Can you work these out from the model? Positions are in its coordinate system, mm. Give positions to 0.01 mm unless a question says otherwise; leave off trailing zeros. Order: outer loops, then holes, each group sorted by start corner. A loop starts at its lowest first (then second) coordinate and runs counter-clockwise, first axis right, second up. Notation, with made-up numbers: (41.25, -16.5) - (75.25, -16.5) arc R24 ccw to (75.25, -6.5) - close; hole circle Ø8 at (-37, -21). An arc over 180 degrees is marked (long way). One line per question, with ' | ' between items.
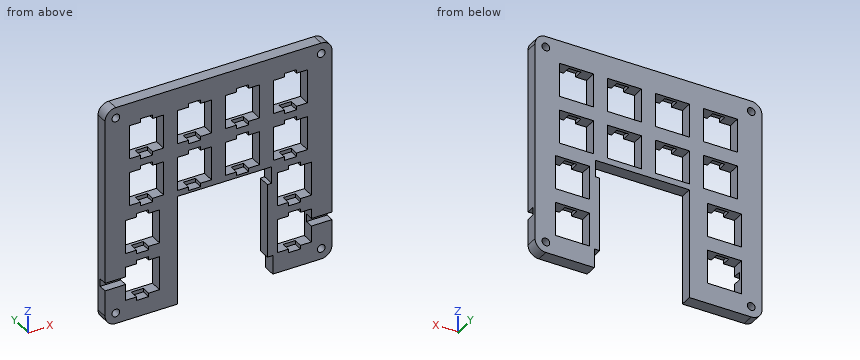
```python
from build123d import *

# Parameters (mm, degrees)
SKETCH2_R           = 1.6
BOSS_EXTRUDE1_DEPTH = 5
CUT_EXTRUDE1_DEPTH  = 3.5
SKETCH4_W           = 2.5
SKETCH4_H           = 1.5
CUT_EXTRUDE2_DEPTH  = 3.7


with BuildPart() as part:
    # Sketch2 → Boss-Extrude1 (new body)
    with BuildSketch(Plane(origin=(0, 0, 0), x_dir=(1, 0, 0), z_dir=(0, 1, 0))):
        with BuildLine():
            Line((-46.858540632, -41.275), (-46.858540632, 41.275))
            ThreePointArc((-46.858540632, 41.275), (-45.557936393, 44.414936393), (-42.418, 45.715540632))
            Line((-42.418, 45.715540632), (-16.875382857, 45.715540632))
            Line((-16.875382857, 45.715540632), (-16.875382857, 30.218907102))
            Line((-16.875382857, 30.218907102), (-16.875382857, 0.094907102))
            Line((-16.875382857, 0.094907102), (-9.912382857, 0.094907102))
            Line((-9.912382857, 0.094907102), (21.96872062, 0.094907102))
            Line((21.96872062, 0.094907102), (21.96872062, 7.075))
            Line((21.96872062, 7.075), (20.16872062, 7.075))
            Line((20.16872062, 7.075), (20.16872062, 9.575))
            Line((20.16872062, 9.575), (20.16872062, 37.797317828))
            Line((20.16872062, 37.797317828), (22.418, 37.797317828))
            Line((22.418, 37.797317828), (22.418, 39.575))
            Line((22.418, 39.575), (22.418, 41.275))
            Line((22.418, 41.275), (22.418, 45.715540632))
            Line((22.418, 45.715540632), (42.418, 45.715540632))
            ThreePointArc((42.418, 45.715540632), (45.557936393, 44.414936393), (46.858540632, 41.275))
            Line((46.858540632, 41.275), (46.858540632, -41.275))
            ThreePointArc((46.858540632, -41.275), (45.557936393, -44.414936393), (42.418, -45.715540632))
            Line((42.418, -45.715540632), (-42.418, -45.715540632))
            ThreePointArc((-42.418, -45.715540632), (-45.557936393, -44.414936393), (-46.858540632, -41.275))
        make_face()
        with Locations(Location((42.418, 41.275, 0), (0, 0, 270))):
            Circle(SKETCH2_R, mode=Mode.SUBTRACT)
        with Locations(Location((-42.418, 41.275, 0), (0, 0, 270))):
            Circle(SKETCH2_R, mode=Mode.SUBTRACT)
        with Locations(Location((-42.418, -41.275, 0), (0, 0, 270))):
            Circle(SKETCH2_R, mode=Mode.SUBTRACT)
        with Locations(Location((42.418, -41.275, 0), (0, 0, 270))):
            Circle(SKETCH2_R, mode=Mode.SUBTRACT)
        Polygon((-31.375382857, 37.218907102), (-38.375382857, 37.218907102), (-38.375382857, 23.218907102), (-24.375382857, 23.218907102), (-24.375382857, 37.218907102), align=None, mode=Mode.SUBTRACT)
        Polygon((-38.375382857, 10.406907102), (-38.375382857, 17.406907102), (-24.375382857, 17.406907102), (-24.375382857, 3.406907102), (-38.375382857, 3.406907102), align=None, mode=Mode.SUBTRACT)
        Polygon((-36.724382857, -9.405092898), (-36.724382857, -2.405092898), (-22.724382857, -2.405092898), (-22.724382857, -16.405092898), (-36.724382857, -16.405092898), align=None, mode=Mode.SUBTRACT)
        Polygon((-36.724382857, -29.217092898), (-36.724382857, -22.217092898), (-22.724382857, -22.217092898), (-22.724382857, -36.217092898), (-36.724382857, -36.217092898), align=None, mode=Mode.SUBTRACT)
        Polygon((-9.912382857, -22.217092898), (-2.912382857, -22.217092898), (-2.912382857, -36.217092898), (-16.912382857, -36.217092898), (-16.912382857, -22.217092898), align=None, mode=Mode.SUBTRACT)
        Polygon((-9.912382857, -16.405092898), (-2.912382857, -16.405092898), (-2.912382857, -2.405092898), (-16.912382857, -2.405092898), (-16.912382857, -16.405092898), align=None, mode=Mode.SUBTRACT)
        Polygon((9.899617143, -2.405092898), (2.899617143, -2.405092898), (2.899617143, -16.405092898), (16.899617143, -16.405092898), (16.899617143, -2.405092898), align=None, mode=Mode.SUBTRACT)
        Polygon((9.899617143, -22.217092898), (2.899617143, -22.217092898), (2.899617143, -36.217092898), (16.899617143, -36.217092898), (16.899617143, -22.217092898), align=None, mode=Mode.SUBTRACT)
        Polygon((36.711617143, -29.217092898), (36.711617143, -22.217092898), (22.711617143, -22.217092898), (22.711617143, -36.217092898), (36.711617143, -36.217092898), align=None, mode=Mode.SUBTRACT)
        Polygon((29.711617143, -2.405092898), (22.711617143, -2.405092898), (22.711617143, -16.405092898), (36.711617143, -16.405092898), (36.711617143, -2.405092898), align=None, mode=Mode.SUBTRACT)
        Polygon((38.362617143, 10.406907102), (38.362617143, 17.406907102), (24.362617143, 17.406907102), (24.362617143, 3.406907102), (38.362617143, 3.406907102), align=None, mode=Mode.SUBTRACT)
        Polygon((38.362617143, 30.218907102), (38.362617143, 23.218907102), (24.362617143, 23.218907102), (24.362617143, 37.218907102), (38.362617143, 37.218907102), align=None, mode=Mode.SUBTRACT)
    extrude(amount=BOSS_EXTRUDE1_DEPTH)

    # Sketch3 → Cut-Extrude1 (cut)
    with BuildSketch(Plane.XZ):
        Polygon((38.362617143, -30.492), (42.418, -30.492), (46.218, -30.492), (46.858540632, -30.492), (46.858540632, -27.292), (46.218, -27.292), (38.362617143, -27.292), align=None)
        Polygon((-46.218, -27.292), (-46.858540632, -27.292), (-46.858540632, -30.492), (-46.218, -30.492), (-42.418, -30.492), (-38.375382857, -30.492), (-38.375382857, -27.292), align=None)
    extrude(amount=-CUT_EXTRUDE1_DEPTH, mode=Mode.SUBTRACT)

    # Sketch4 → Cut-Extrude2 (cut)
    with BuildSketch(Plane.XZ):
        with Locations((32.612617143, -37.968907102)):
            Rectangle(SKETCH4_W, SKETCH4_H)
        with Locations((30.112617143, -37.968907102)):
            Rectangle(SKETCH4_W, SKETCH4_H)
        with Locations((32.612617143, -22.468907102)):
            Rectangle(SKETCH4_W, SKETCH4_H)
        with Locations((30.112617143, -22.468907102)):
            Rectangle(SKETCH4_W, SKETCH4_H)
        with Locations((32.612617143, -2.656907102)):
            Rectangle(SKETCH4_W, SKETCH4_H)
        with Locations((30.112617143, -18.156907102)):
            Rectangle(SKETCH4_W, SKETCH4_H)
        with Locations((32.612617143, -18.156907102)):
            Rectangle(SKETCH4_W, SKETCH4_H)
        with Locations((30.112617143, -2.656907102)):
            Rectangle(SKETCH4_W, SKETCH4_H)
        with Locations((30.961617143, 1.655092898)):
            Rectangle(SKETCH4_W, SKETCH4_H)
        with Locations((28.461617143, 1.655092898)):
            Rectangle(SKETCH4_W, SKETCH4_H)
        with Locations((30.961617143, 17.155092898)):
            Rectangle(SKETCH4_W, SKETCH4_H)
        with Locations((28.461617143, 17.155092898)):
            Rectangle(SKETCH4_W, SKETCH4_H)
        with Locations((30.961617143, 21.467092898)):
            Rectangle(SKETCH4_W, SKETCH4_H)
        with Locations((28.461617143, 21.467092898)):
            Rectangle(SKETCH4_W, SKETCH4_H)
        with Locations((30.961617143, 36.967092898)):
            Rectangle(SKETCH4_W, SKETCH4_H)
        with Locations((28.461617143, 36.967092898)):
            Rectangle(SKETCH4_W, SKETCH4_H)
        with Locations((11.149617143, 36.967092898)):
            Rectangle(SKETCH4_W, SKETCH4_H)
        with Locations((8.649617143, 36.967092898)):
            Rectangle(SKETCH4_W, SKETCH4_H)
        with Locations((8.649617143, 21.467092898)):
            Rectangle(SKETCH4_W, SKETCH4_H)
        with Locations((11.149617143, 21.467092898)):
            Rectangle(SKETCH4_W, SKETCH4_H)
        with Locations((11.149617143, 17.155092898)):
            Rectangle(SKETCH4_W, SKETCH4_H)
        with Locations((8.649617143, 17.155092898)):
            Rectangle(SKETCH4_W, SKETCH4_H)
        with Locations((11.149617143, 1.655092898)):
            Rectangle(SKETCH4_W, SKETCH4_H)
        with Locations((8.649617143, 1.655092898)):
            Rectangle(SKETCH4_W, SKETCH4_H)
        with Locations((-8.662382857, 1.655092898)):
            Rectangle(SKETCH4_W, SKETCH4_H)
        with Locations((-11.162382857, 1.655092898)):
            Rectangle(SKETCH4_W, SKETCH4_H)
        with Locations((-8.662382857, 17.155092898)):
            Rectangle(SKETCH4_W, SKETCH4_H)
        with Locations((-11.162382857, 17.155092898)):
            Rectangle(SKETCH4_W, SKETCH4_H)
        with Locations((-8.662382857, 21.467092898)):
            Rectangle(SKETCH4_W, SKETCH4_H)
        with Locations((-11.162382857, 21.467092898)):
            Rectangle(SKETCH4_W, SKETCH4_H)
        with Locations((-8.662382857, 36.967092898)):
            Rectangle(SKETCH4_W, SKETCH4_H)
        with Locations((-11.162382857, 36.967092898)):
            Rectangle(SKETCH4_W, SKETCH4_H)
        with Locations((-28.474382857, 17.155092898)):
            Rectangle(SKETCH4_W, SKETCH4_H)
        with Locations((-30.974382857, 17.155092898)):
            Rectangle(SKETCH4_W, SKETCH4_H)
        with Locations((-30.974382857, 21.467092898)):
            Rectangle(SKETCH4_W, SKETCH4_H)
        with Locations((-28.474382857, 21.467092898)):
            Rectangle(SKETCH4_W, SKETCH4_H)
        with Locations((-28.474382857, 36.967092898)):
            Rectangle(SKETCH4_W, SKETCH4_H)
        with Locations((-30.974382857, 36.967092898)):
            Rectangle(SKETCH4_W, SKETCH4_H)
        with Locations((-28.474382857, 1.655092898)):
            Rectangle(SKETCH4_W, SKETCH4_H)
        with Locations((-30.974382857, 1.655092898)):
            Rectangle(SKETCH4_W, SKETCH4_H)
        Polygon((-33.875382857, -1.906907102), (-33.875382857, -3.406907102), (-31.375382857, -3.406907102), (-28.875382857, -3.406907102), (-28.875382857, -1.906907102), align=None)
        with Locations((-32.625382857, -18.156907102)):
            Rectangle(SKETCH4_W, SKETCH4_H)
        with Locations((-30.125382857, -18.156907102)):
            Rectangle(SKETCH4_W, SKETCH4_H)
        with Locations((-32.625382857, -22.468907102)):
            Rectangle(SKETCH4_W, SKETCH4_H)
        with Locations((-30.125382857, -22.468907102)):
            Rectangle(SKETCH4_W, SKETCH4_H)
        with Locations((-30.125382857, -37.968907102)):
            Rectangle(SKETCH4_W, SKETCH4_H)
        with Locations((-32.625382857, -37.968907102)):
            Rectangle(SKETCH4_W, SKETCH4_H)
    extrude(amount=-CUT_EXTRUDE2_DEPTH, mode=Mode.SUBTRACT)


solid = part.part
```
(1) Imagine slicing it at A-A (x = 14). List the corners of the cut face in (y, z) for me.
Answer below:
outline: (0, -0.09) - (5, -0.09) - (5, 2.41) - (0, 2.41) - close; (0, 16.41) - (5, 16.41) - (5, 22.22) - (0, 22.22) - close; (0, 36.22) - (5, 36.22) - (5, 45.72) - (0, 45.72) - close
(2) Imagine slicing it at C-C (z = -35). List the corners of the cut face in (x, y) for me.
Answer below:
outline: (-46.86, 0) - (-38.38, 0) - (-38.38, 5) - (-46.86, 5) - close; (-24.38, 0) - (-16.88, 0) - (-16.88, 5) - (-24.38, 5) - close; (20.17, 0) - (24.36, 0) - (24.36, 5) - (20.17, 5) - close; (38.36, 0) - (46.86, 0) - (46.86, 5) - (38.36, 5) - close
(3) Imagine slicing it at D-D (y = 1.9). Count the separate pieces of the cut face and the enclosed holes in it, and give its area (3 significant figures).
Answer below:
separate pieces: 1 | enclosed holes: 14 | area: 4,210 mm^2
(4) If I drill on line 1 (Z direction, x = 11.5, y = 2); line 2 (Z direction, x = -10, y = 4.85); line 3 (X direction, y = 0.6, z = -24), over which ranges is the centre line in solid material (lowest first)?
Answer below:
line 1: -0.09 to 0.91, 17.91 to 20.72, 37.72 to 45.72 | line 2: -0.09 to 2.41, 16.41 to 22.22, 36.22 to 45.72 | line 3: -46.86 to -38.38, -24.38 to -16.88, 20.17 to 24.36, 38.36 to 46.86
(5) Imagine slicing it at B-B (z = 8). List the corners of the cut face in (x, y) for me.
Answer below:
outline: (-46.86, 0) - (-36.72, 0) - (-36.72, 5) - (-46.86, 5) - close; (-22.72, 0) - (-16.91, 0) - (-16.91, 5) - (-22.72, 5) - close; (-2.91, 0) - (2.9, 0) - (2.9, 5) - (-2.91, 5) - close; (16.9, 0) - (22.71, 0) - (22.71, 5) - (16.9, 5) - close; (36.71, 0) - (46.86, 0) - (46.86, 5) - (36.71, 5) - close
(6) Will these pins go through, and if not, where does the flat tip stop? pin 1 (1.5 mm diameter, centred on x = 4.5, y = 2.5, fed in from -Z); pin 2 (0.8 mm diameter, centred on x = 11, z = 1.5, fed in from -Y); pin 3 (1.2 mm diameter, centred on x = -29.5, z = 17.5, fed in from -Y).
Answer below:
pin 1: z = -0.09 | pin 2: y = 3.7 | pin 3: y = 0
